Could you check a few things on this model? Use its own coordinates, in mm. Face numbers are marked on the shaded views. A direction names the side the tool comes from. Give positions to 0.01 mm unless a question says otherwise; leave off trailing zeros. Write each loop counter-clockwise with the first axis right and the second up, starting at its lowest first coordinate (ties: lowest second). Pieces come first, ordered by that corner, then holes. Notation, with made-up numbers: (45.25, 66.25) -> (76.25, 66.25) arc R13 cw to (76.25, 73.25) -> close; hole circle Ø5 at (-38.5, -22.75). An arc over 180 degrees is marked (long way). Write item = value, one per line. Start each with the question number.
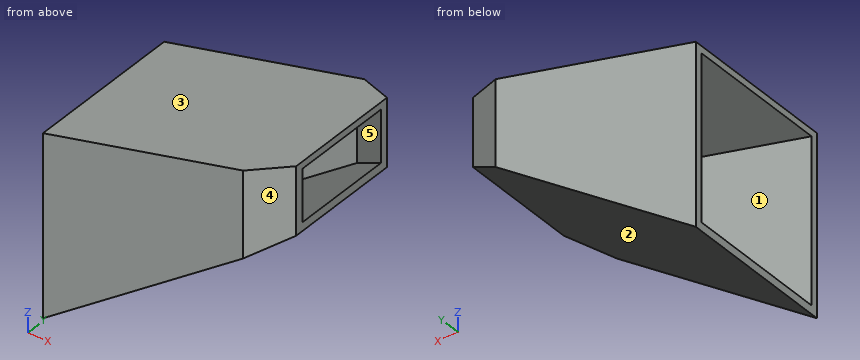
```python
from build123d import *

# Parameters (mm, degrees)
BOSS_EXTRUDE1_DEPTH = 40
CHAMFER1_SIZE       = 5
CHAMFER1_SIZE2      = 10
CHAMFER2_SIZE       = 10
CHAMFER2_SIZE2      = 5
SHELL1_T            = -1.8


with BuildPart() as part:
    # Sketch2 → Boss-Extrude1 (new body)
    with BuildSketch(Plane(origin=(0, 0, 0), x_dir=(1, 0, 0), z_dir=(0, 1, 0))):
        Polygon((13.428152071, -6.099992503), (13.428152071, 41.830007497), (76.327388482, -6.373909949), (76.327388482, -24.373909949), align=None)
    extrude(amount=BOSS_EXTRUDE1_DEPTH)

    # Chamfer1
    chamfer1_edges = [part.edges().sort_by_distance(p)[0] for p in [
        (76.327388482, 40, 15.373909949),
    ]]
    chamfer1_side = [part.faces().sort_by_distance(p)[0] for p in [
        (76.327388482, 20, 15.373909949),
    ]]
    chamfer(chamfer1_edges, length=CHAMFER1_SIZE, length2=CHAMFER1_SIZE2, reference=chamfer1_side[0])

    # Chamfer2
    chamfer2_edges = [part.edges().sort_by_distance(p)[0] for p in [
        (76.327388482, 0, 15.373909949),
    ]]
    chamfer2_side = [part.faces().sort_by_distance(p)[0] for p in [
        (40.118747713, 0, -3.760440323),
    ]]
    chamfer(chamfer2_edges, length=CHAMFER2_SIZE, length2=CHAMFER2_SIZE2, reference=chamfer2_side[0])

    # Shell1
    shell1_openings = [part.faces().sort_by_distance(p)[0] for p in [
        (13.428152071, 20, -17.865007497),
        (76.327388482, 20, 15.373909949),
    ]]
    offset(amount=SHELL1_T, openings=shell1_openings, kind=Kind.INTERSECTION)


solid = part.part
```
(1) On a 3-axis mill with a long thin cutter (end or side, diameter ignored), from which of +Z, -Z, +X, -X, +Y, -Y can I reach the whole of each face in a straight line? I mean the marked faces 4 and 5. Say none if no direction works.
(2) Imagine slicing it at B-B (x = 72.5). Please give me the cut outline in (y, z), then the cut area to 3 significant figures.
(3) We'd pull the mould along X, two halves only. Please class the marked faces 1, 2 and 3: released by +X, released by -X, zero draft, split by the parting line, or undercut.
(4) If I drill on line 1 along Y through (x, z) = (23.5, -29.5); line 2 along Z through (x, y) = (41.5, 7); line 3 along Z through (x, y) = (20, 38), over which ranges is the centre line in solid material (lowest first)? Write a range as from..to.
(5) Imagine slicing it at A-A (y = 15). Please give me the cut outline in (x, z), then the cut area to 3 significant figures.
(6) Imagine slicing it at D-D (x = 30). Please give me the cut outline in (y, z), then the cut area to 3 significant figures.
(7) I'm going to push flat-ended pins straight in: pin 1 (4 mm diameter, centred on y = 5.5, z = -33.5, fed in from -X); pin 2 (2 mm diameter, centred on x = 30.5, y = 7.5, fed in from +Z); pin 3 (1.5 mm diameter, centred on x = 30.5, y = 7.5, fed in from +Z). Where does each tip first touch, or does it pass through?
(8) Imagine slicing it at C-C (z = 18). Please give me the cut outline in (x, y), then the cut area to 3 significant figures.
Answers below:
q1.face_4 = +Z, -Z, +X, -Y
q1.face_5 = none
q2.outline = (3.09, 3.44) -> (36.91, 3.44) -> (36.91, 23.26) -> (3.09, 23.26) -> close; hole (5.1, 5.71) -> (34.9, 5.71) -> (34.9, 21.39) -> (5.1, 21.39) -> close
q2.area = 203 mm^2
q3.face_1 = undercut
q3.face_2 = released by +X
q3.face_3 = released by -X
q4.line_1 = 0..1.8, 38.2..40
q4.line_2 = -20.32..-18.05, 12.38..14.26
q4.line_3 = -36.79..-34.53, 6.13..8.01
q5.outline = (13.43, -41.83) -> (76.33, 6.37) -> (76.33, 8.64) -> (13.43, -39.56) -> close; (13.43, 4.23) -> (76.33, 22.5) -> (76.33, 24.37) -> (13.43, 6.1) -> close
q5.area = 261 mm^2
q6.outline = (0, -29.13) -> (40, -29.13) -> (40, 10.91) -> (0, 10.91) -> close; hole (1.8, -26.86) -> (38.2, -26.86) -> (38.2, 9.04) -> (1.8, 9.04) -> close
q6.area = 295 mm^2
q7.pin_1 = 18.73
q7.pin_2 = 11.35
q7.pin_3 = 11.28
q8.outline = (54.39, 0) -> (66.33, 0) -> (76.33, 5) -> (76.33, 7.01) -> (65.9, 1.8) -> (60.84, 1.8) -> (60.84, 38.2) -> (65.9, 38.2) -> (76.33, 32.99) -> (76.33, 35) -> (66.33, 40) -> (54.39, 40) -> close
q8.area = 318 mm^2
